Input: part model. Units: mm. Frame: model coordinates. A direction names the side the tool comes from. Give positions to 0.01 mm unless a question says otherwise; leave off trailing zeros. Loops run counter-clockwise (first coordinate to the right, second up) from the corner with the lowest first, then second, coordinate; pieces in that order, holes last.
from build123d import *

# Parameters (mm, degrees)
SKETCH_1_W             = 80
SKETCH_1_H             = 80
EXTRUDE_1_DEPTH        = 6.5
FILLET_1_R             = 10
SKETCH_55_R            = 1.5
CUT_EXTRUDE_33_DEPTH   = 10
SKETCH_57_R            = 3.5
CUT_EXTRUDE_34_DEPTH   = 3.5
SKETCH_58_W            = 7.18
SKETCH_58_H            = 5
CUT_EXTRUDE_35_DEPTH   = 7.5
SKETCH_60_R            = 1.6
CUT_EXTRUDE_36_DEPTH   = 10
SKETCH_61_R            = 3.15
CUT_EXTRUDE_37_DEPTH   = 3
SKETCH_62_W            = 7.18
SKETCH_62_H            = 4
EXTRUDE_8_DEPTH        = 25
FILLET_8_R             = 5
CUT_EXTRUDE_38_DEPTH   = 25
FILLET_9_R             = 2
FILLET_8_OF_MIRROR_1_R = 5
FILLET_9_OF_MIRROR_1_R = 2


with BuildPart() as part:
    # 草图1 → 凸台-拉伸1 (new body)
    with BuildSketch(Plane(origin=(0, 0, 0), x_dir=(1, 0, 0), z_dir=(0, 1, 0))):
        Rectangle(SKETCH_1_W, SKETCH_1_H)
    extrude(amount=EXTRUDE_1_DEPTH)

    # 圆角1
    fillet_1_edges = [part.edges().sort_by_distance(p)[0] for p in [
        (40, 3.25, 40),
        (-40, 3.25, 40),
        (-40, 3.25, -40),
        (40, 3.25, -40),
    ]]
    fillet(fillet_1_edges, radius=FILLET_1_R)

    # 草图55 → 切除-拉伸33 (cut)
    with BuildSketch(Plane(origin=(0, 6.5, 0), x_dir=(1, 0, 0), z_dir=(0, 1, 0))):
        with Locations(Location((-7, -12.124355653, 0), (0, 0, 270))):
            Circle(SKETCH_55_R)
        with Locations(Location((-14, 0, 0), (0, 0, 270))):
            Circle(SKETCH_55_R)
        with Locations(Location((-7, 12.124355653, 0), (0, 0, 270))):
            Circle(SKETCH_55_R)
        with Locations(Location((7, 12.124355653, 0), (0, 0, 270))):
            Circle(SKETCH_55_R)
        with Locations(Location((7, -12.124355653, 0), (0, 0, 270))):
            Circle(SKETCH_55_R)
        with Locations(Location((14, 0, 0), (0, 0, 270))):
            Circle(SKETCH_55_R)
    extrude(amount=-CUT_EXTRUDE_33_DEPTH, mode=Mode.SUBTRACT)

    # 草图57 → 切除-拉伸34 (cut)
    with BuildSketch(Plane(origin=(0, 6.5, 0), x_dir=(1, 0, 0), z_dir=(0, 1, 0))):
        with Locations(Location((14, 0, 0), (0, 0, 270))):
            Circle(SKETCH_57_R)
        with Locations(Location((7, -12.124355653, 0), (0, 0, 270))):
            Circle(SKETCH_57_R)
        with Locations(Location((-7, -12.124355653, 0), (0, 0, 270))):
            Circle(SKETCH_57_R)
        with Locations(Location((-14, 0, 0), (0, 0, 270))):
            Circle(SKETCH_57_R)
        with Locations(Location((-7, 12.124355653, 0), (0, 0, 270))):
            Circle(SKETCH_57_R)
        with Locations(Location((7, 12.124355653, 0), (0, 0, 270))):
            Circle(SKETCH_57_R)
    extrude(amount=-CUT_EXTRUDE_34_DEPTH, mode=Mode.SUBTRACT)

    # 草图58 → 切除-拉伸35 (cut)
    with BuildSketch(Plane(origin=(0, 6.5, 0), x_dir=(1, 0, 0), z_dir=(0, 1, 0))):
        with Locations((-28.500986742, -30.1)):
            Rectangle(SKETCH_58_W, SKETCH_58_H)
        with Locations((-28.500986742, 30.1)):
            Rectangle(SKETCH_58_W, SKETCH_58_H)
    extrude(amount=-CUT_EXTRUDE_35_DEPTH, mode=Mode.SUBTRACT)

    # 草图60 → 切除-拉伸36 (cut)
    with BuildSketch(Plane(origin=(0, 6.5, 0), x_dir=(1, 0, 0), z_dir=(0, 1, 0))):
        with Locations(Location((-36, -15, 0), (0, 0, 270))):
            Circle(SKETCH_60_R)
        with Locations(Location((-36, 15, 0), (0, 0, 270))):
            Circle(SKETCH_60_R)
        with Locations(Location((33, -28, 0), (0, 0, 270))):
            Circle(SKETCH_60_R)
        with Locations(Location((33, 28, 0), (0, 0, 270))):
            Circle(SKETCH_60_R)
    extrude(amount=-CUT_EXTRUDE_36_DEPTH, mode=Mode.SUBTRACT)

    # 草图61 → 切除-拉伸37 (cut)
    with BuildSketch(Plane.XZ):
        with Locations(Location((-36, 15, 0), (0, 0, 270))):
            Circle(SKETCH_61_R)
        with Locations(Location((-36, -15, 0), (0, 0, 270))):
            Circle(SKETCH_61_R)
        with Locations(Location((33, -28, 0), (0, 0, 270))):
            Circle(SKETCH_61_R)
        with Locations(Location((33, 28, 0), (0, 0, 270))):
            Circle(SKETCH_61_R)
    extrude(amount=-CUT_EXTRUDE_37_DEPTH, mode=Mode.SUBTRACT)

    # 草图62 → 凸台-拉伸8 (add)
    with BuildSketch(Plane(origin=(0, 6.5, 0), x_dir=(1, 0, 0), z_dir=(0, 1, 0))):
        with Locations((-28.500986742, 25.6)):
            Rectangle(SKETCH_62_W, SKETCH_62_H)
    extrude_8 = extrude(amount=EXTRUDE_8_DEPTH)

    # 圆角8
    fillet_8_edges = [part.edges().sort_by_distance(p)[0] for p in [
        (-32.090986742, 6.5, -25.6),
        (-24.910986742, 6.5, -25.6),
    ]]
    fillet(fillet_8_edges, radius=FILLET_8_R)

    # 草图63 → 切除-拉伸38 (cut)
    with BuildSketch(Plane(origin=(0, 0, -27.6), x_dir=(-1, 0, 0), z_dir=(0, 0, -1))):
        with BuildLine():
            Line((29.600986742, 29.313400897), (29.600986742, 9.313400897))
            ThreePointArc((29.600986742, 9.313400897), (28.500986742, 8.213400897), (27.400986742, 9.313400897))
            Line((27.400986742, 9.313400897), (27.400986742, 29.313400897))
            ThreePointArc((27.400986742, 29.313400897), (28.500986742, 30.413400897), (29.600986742, 29.313400897))
        make_face()
    cut_extrude_38 = extrude(amount=-CUT_EXTRUDE_38_DEPTH, mode=Mode.SUBTRACT)

    # 圆角9
    fillet_9_edges = [part.edges().sort_by_distance(p)[0] for p in [
        (-32.090986742, 31.5, -25.6),
        (-24.910986742, 31.5, -25.6),
    ]]
    fillet(fillet_9_edges, radius=FILLET_9_R)

    # 镜向1: 凸台-拉伸8, 切除-拉伸38 across plane
    add(extrude_8.mirror(Plane.XY))
    add(cut_extrude_38.mirror(Plane.XY), mode=Mode.SUBTRACT)

    # 圆角8 of 镜向1
    fillet_8_of_mirror_1_edges = [part.edges().sort_by_distance(p)[0] for p in [
        (-32.090986742, 6.5, 25.6),
        (-24.910986742, 6.5, 25.6),
    ]]
    fillet(fillet_8_of_mirror_1_edges, radius=FILLET_8_OF_MIRROR_1_R)

    # 圆角9 of 镜向1
    fillet_9_of_mirror_1_edges = [part.edges().sort_by_distance(p)[0] for p in [
        (-32.090986742, 31.5, 25.6),
        (-24.910986742, 31.5, 25.6),
    ]]
    fillet(fillet_9_of_mirror_1_edges, radius=FILLET_9_OF_MIRROR_1_R)


solid = part.part
(1) Ray query, probe 1 along X at (y, z) = (1.4, 28); probe 2 along X at (y, z) = (25.5, 24.5); probe 3 along Y at (x, z) = (-8, -25). Return the intervals inside material, ascending.
Values follow:
probe 1: x = -40 to -32.09, -24.91 to 29.85, 36.15 to 40
probe 2: x = -32.09 to -29.6, -27.4 to -24.91
probe 3: y = 0 to 6.5
(2) Pin query (flat end, axial travel): pin 1 Ø1.8 at (x, z) = (-7, -12.12) entering from -Y; pin 2 Ø2 at (y, z) = (21, -26) entering from -X; pin 3 Ø5 at (x, z) = (33, 28) entering from -Y; pin 4 Ø6 at (x, y) = (-28.5, 24) entering from -Z. Return the tip coordinate at first contact, or that it passes through.
Values follow:
pin 1: passes through
pin 2: stops at x = -32.09
pin 3: stops at y = 3
pin 4: stops at z = -27.6
(3) Cut plane B-B (x = -14). Return the cut outline in (y, z), and give its area (4 significant figures).
Values follow:
outline: (0, -40) - (6.5, -40) - (6.5, -3.5) - (3, -3.5) - (3, -1.5) - (0, -1.5) - close; (0, 1.5) - (3, 1.5) - (3, 3.5) - (6.5, 3.5) - (6.5, 40) - (0, 40) - close
area: 486.5 mm2
(4) Mould query, pull axis Z, two halves, no side actions, for faces 5 (the flat face through (-27, 15, 27.6)), 6 (the cylindrical face through (-23.41, 7.93, -25.63)), 7 (the cylindrical face through (-37.15, 3.3, -36.99)). Classes: +Z half, -Z half, draft (parallel to the pull), parting line (faces both ways), or undercut.
Values follow:
face 5: undercut
face 6: draft
face 7: -Z half
(5) Cut plane A-A (y = 27). Return the cut outline in (x, z), and give its area (3 significant figures).
Values follow:
outline: (-32.09, -27.6) - (-29.6, -27.6) - (-29.6, -23.6) - (-32.09, -23.6) - close; (-32.09, 23.6) - (-29.6, 23.6) - (-29.6, 27.6) - (-32.09, 27.6) - close; (-27.4, -27.6) - (-24.91, -27.6) - (-24.91, -23.6) - (-27.4, -23.6) - close; (-27.4, 23.6) - (-24.91, 23.6) - (-24.91, 27.6) - (-27.4, 27.6) - close
area: 39.8 mm2
(6) Cut plane C-C (z = 0). Return the cut outline in (x, y).
Values follow:
outline: (-40, 0) - (-15.5, 0) - (-15.5, 3) - (-17.5, 3) - (-17.5, 6.5) - (-40, 6.5) - close; (-12.5, 0) - (12.5, 0) - (12.5, 3) - (10.5, 3) - (10.5, 6.5) - (-10.5, 6.5) - (-10.5, 3) - (-12.5, 3) - close; (15.5, 0) - (40, 0) - (40, 6.5) - (17.5, 6.5) - (17.5, 3) - (15.5, 3) - close
(7) Cut plane D-D (x = 7). Return the cut outline in (y, z), and give its area (3 significant figures).
Values follow:
outline: (0, -40) - (6.5, -40) - (6.5, -15.62) - (3, -15.62) - (3, -13.62) - (0, -13.62) - close; (0, -10.62) - (3, -10.62) - (3, -8.62) - (6.5, -8.62) - (6.5, 8.62) - (3, 8.62) - (3, 10.62) - (0, 10.62) - close; (0, 13.62) - (3, 13.62) - (3, 15.62) - (6.5, 15.62) - (6.5, 40) - (0, 40) - close
area: 453 mm2
(8) Reachability of faces 1 (the cylindrical face through (-28.525, 8.214, -25.628)), 2 (the flat face through (-32.091, 3, 30)), 3 (the flat face through (-14, 3, 2)), 4 (the flat face through (-32.091, 20, 26)) from +Z, -Z, +X, -X, +Y, -Y: full face, straight path, thin tool, end or side. Return the list, or none.
Values follow:
face 1: +Z, -Z
face 2: +Y, -Y
face 3: +Y
face 4: +Z, -Z, -X, +Y
